Verification items for this drawing (mm, ordinates from the low corner). A direction names the side the tool comes from. Round coordinates to 2 decimals unless told otherwise and drop trailing zeros. Loops run counter-clockwise (first coordinate to the right, second up) from the corner with the lowest first, then second, coordinate; pieces in that order, holes last. Notation, with made-up numbers: (69.5, -7) - (82.5, -7) arc R19 cw to (82.5, 7) - close; hole circle Ø3 at (26, -32.5). An arc over 180 degrees is marked (long way). Use a Markdown table: item, result. Add a question column.
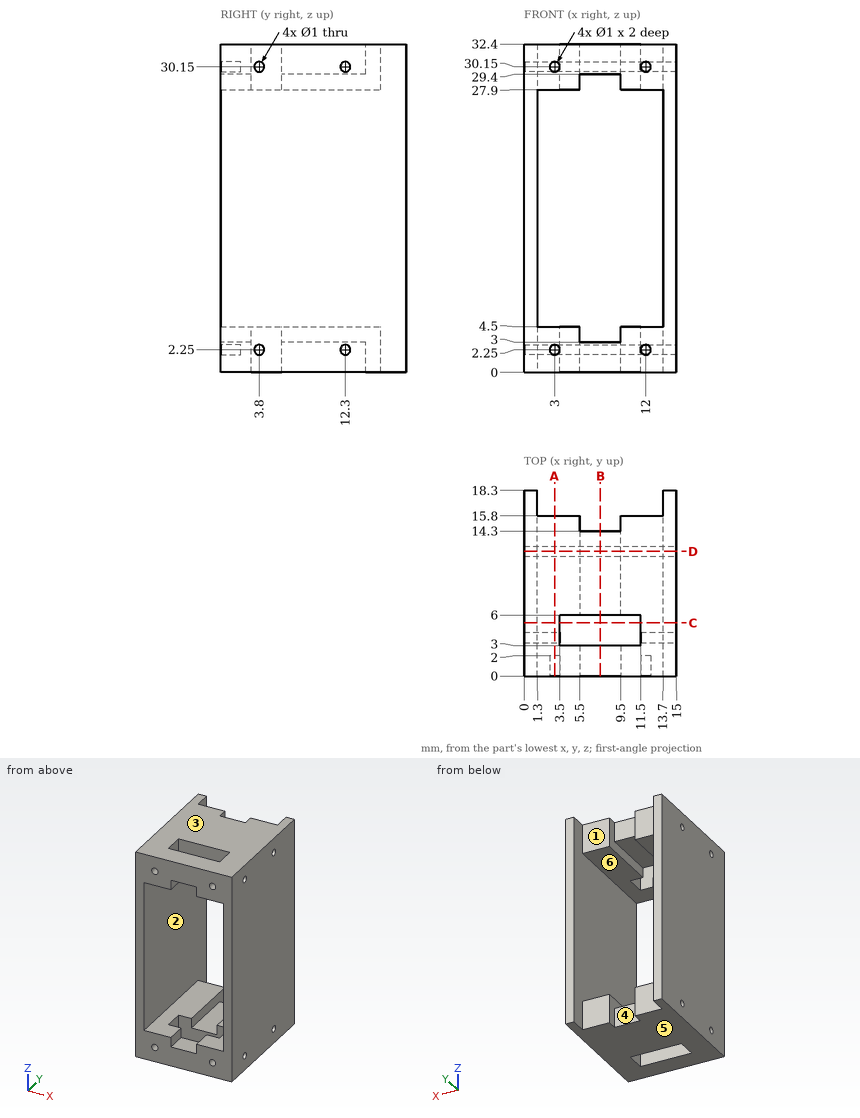
Q1. Section check B-B on x = 7.5. Record the cut outline in (y, z).
Q2. Section check D-D on y = 12.3. Record the cut outline in (x, z).
Q3. Set-up check for the marked faces 4, 5 and 6: record each of +Z, -Z, +X, -X, +Y, -Y from which the full face is reachable in a straight line by a thin tool's end or side.
Q4. Thickness scan on line 1 along Y through (x, z) = (2.4, 30.15); line 2 along X through (y, z) = (6.25, 9); line 3 along X through (y, z) = (0.75, 2.25). Record the ranges inside material, lowest first.
Q5. Section check A-A on x = 3. Record the cut outline in (y, z), plus the area to 3 significant figures.
Q6. Go/stop test with flat-tipped pins: pin 1 Ø1.3 at (x, z) = (6, 3) entering from +Y; pin 2 Ø0.9 at (x, z) = (6.5, 31.5) entering from +Y. Record where each tip stops, or that it passes through.
Q7. Release check for a two-part mould opening along Z. For the marked faces 1, 2 and 3 record: +Z half, -Z half, draft (parallel to the pull), parting line (faces both ways), or undercut.
Q8. Section check C-C on y = 5.25. Record the cut outline in (x, z), plus the area to 3 significant figures.
Determined:
| question | item | result |
|---|---|---|
| 1 | outline | (0, 0) - (3, 0) - (3, 3) - (0, 3) - close; (0, 29.4) - (3, 29.4) - (3, 32.4) - (0, 32.4) - close; (6, 0) - (14.3, 0) - (14.3, 3) - (6, 3) - close; (6, 29.4) - (14.3, 29.4) - (14.3, 32.4) - (6, 32.4) - close; hole circle Ø1 at (12.3, 2.25); hole circle Ø1 at (12.3, 30.15) |
| 2 | outline | (0, 0) - (15, 0) - (15, 1.75) - (0, 1.75) - close; (0, 2.75) - (15, 2.75) - (15, 29.65) - (0, 29.65) - close; (0, 30.65) - (15, 30.65) - (15, 32.4) - (0, 32.4) - close; hole (1.3, 4.5) - (5.5, 4.5) - (5.5, 3) - (9.5, 3) - (9.5, 4.5) - (13.7, 4.5) - (13.7, 27.9) - (9.5, 27.9) - (9.5, 29.4) - (5.5, 29.4) - (5.5, 27.9) - (1.3, 27.9) - close |
| 3 | face 4 | +Z, -Z, +Y |
| 3 | face 5 | -Z, +X, -X, +Y, -Y |
| 3 | face 6 | +Y, -Y |
| 4 | line 1 | y = 0 to 3.3, 4.3 to 11.8, 12.8 to 15.8 |
| 4 | line 2 | x = 0 to 1.3, 13.7 to 15 |
| 4 | line 3 | x = 0 to 2.5, 3.5 to 11.5, 12.5 to 15 |
| 5 | outline | (0, 0) - (15.8, 0) - (15.8, 4.5) - (0, 4.5) - (0, 2.75) - (2, 2.75) - (2, 1.75) - (0, 1.75) - close; (0, 27.9) - (15.8, 27.9) - (15.8, 32.4) - (0, 32.4) - (0, 30.65) - (2, 30.65) - (2, 29.65) - (0, 29.65) - close; hole circle Ø1 at (3.8, 2.25); hole circle Ø1 at (3.8, 30.15); hole circle Ø1 at (12.3, 2.25); hole circle Ø1 at (12.3, 30.15) |
| 5 | area | 135 mm² |
| 6 | pin 1 | stops at y = 15.8 |
| 6 | pin 2 | stops at y = 14.3 |
| 7 | face 1 | draft |
| 7 | face 2 | undercut |
| 7 | face 3 | +Z half |
| 8 | outline | (0, 0) - (3.5, 0) - (3.5, 4.5) - (1.3, 4.5) - (1.3, 27.9) - (3.5, 27.9) - (3.5, 32.4) - (0, 32.4) - close; (11.5, 0) - (15, 0) - (15, 32.4) - (11.5, 32.4) - (11.5, 27.9) - (13.7, 27.9) - (13.7, 4.5) - (11.5, 4.5) - close |
| 8 | area | 124 mm² |
